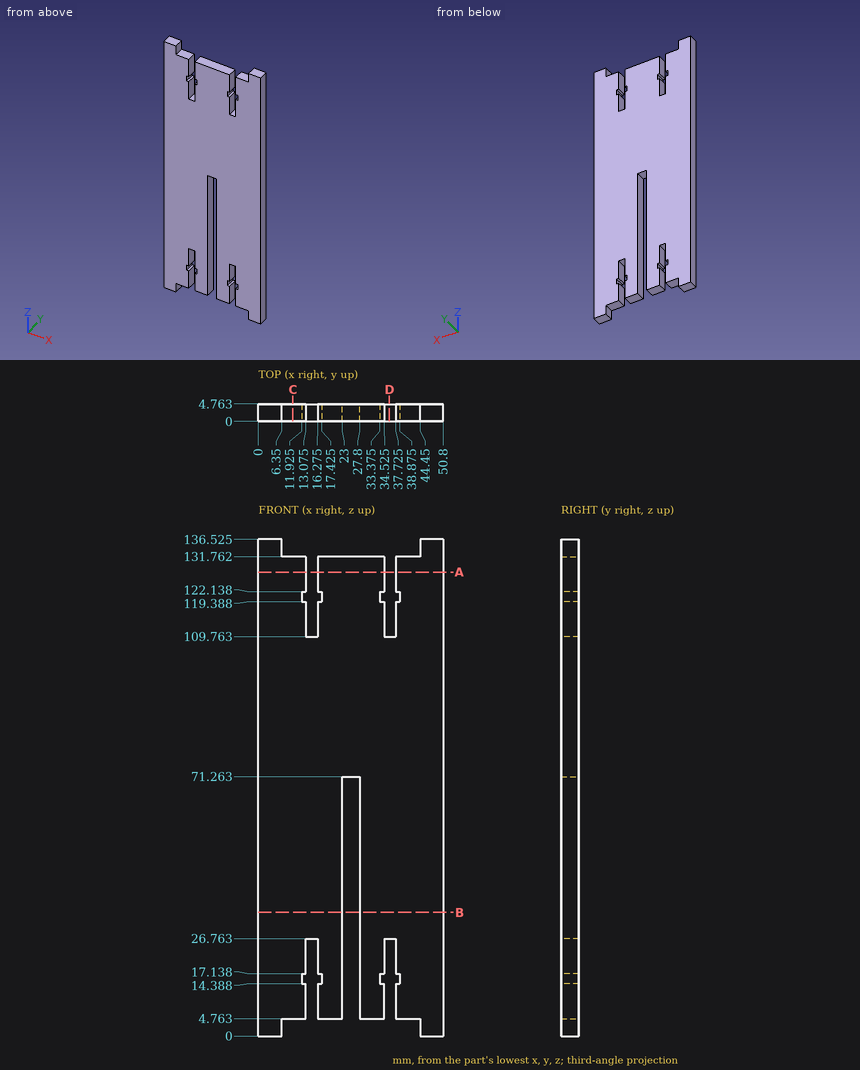
Could you check a few things on this drawing? It's one solid part, dimensions in mm from its lowest x, y, z. Give positions to 0.01 mm unless a question says otherwise; leave off trailing zeros. Order: outer loops, then holes, each group sorted by start corner. A loop starts at its lowest first (then second) coordinate and runs counter-clockwise, first axis right, second up. Notation, with made-up numbers: (-20.5, 66) - (15.5, 66) arc R23 ccw to (15.5, 98) - close; hole circle Ø5 at (51.5, 12.5). An arc over 180 degrees is marked (long way). One line per item, written item: value. Start each with the question number.
1. Imagine slicing it at D-D on x = 36. List the corners of the cut face in (y, z) for me, plus the area to 3 significant figures.
2. For P1, Ø1, axis at x = 8, y = 2.5, coming from the +Z side; P2, Ø0.9, axis at x = 34, y = 3.5, coming from the -Z side; P3, Ø1.6, axis at x = 36, y = 3, coming from the -Z side, each with a flat end and sliding along its axis, tell me the tip position at first contact or that it passes through.
3. Imagine slicing it at C-C on x = 9.5. List the corners of the cut face in (y, z) for me, plus the area to 3 significant figures.
4. Imagine slicing it at B-B on z = 34. List the corners of the cut face in (x, y) for me.
5. If I drill on probe 1 along X at (y, z) = (1.1, 15) (1 decimal); probe 2 along X at (y, z) = (3.8, 118.5) (1 decimal); probe 3 along X at (y, z) = (1.1, 10.5) (1 decimal), over which ranges is the centre line in solid material (lowest first)?
6. Imagine slicing it at A-A on z = 127.5. List the corners of the cut face in (x, y) for me (1 decimal).
Values:
1. outline: (0, 26.76) - (4.76, 26.76) - (4.76, 109.76) - (0, 109.76) - close
1. area: 395 mm²
2. P1: z = 131.76
2. P2: z = 4.76
2. P3: z = 26.76
3. outline: (0, 4.76) - (4.76, 4.76) - (4.76, 131.76) - (0, 131.76) - close
3. area: 605 mm²
4. outline: (0, 0) - (23, 0) - (23, 4.76) - (0, 4.76) - close; (27.8, 0) - (50.8, 0) - (50.8, 4.76) - (27.8, 4.76) - close
5. probe 1: 0 to 11.9, 17.4 to 23, 27.8 to 33.4, 38.9 to 50.8
5. probe 2: 0 to 13.1, 16.3 to 34.5, 37.7 to 50.8
5. probe 3: 0 to 13.1, 16.3 to 23, 27.8 to 34.5, 37.7 to 50.8
6. outline: (0, 0) - (13.1, 0) - (13.1, 4.8) - (0, 4.8) - close; (16.3, 0) - (34.5, 0) - (34.5, 4.8) - (16.3, 4.8) - close; (37.7, 0) - (50.8, 0) - (50.8, 4.8) - (37.7, 4.8) - close
